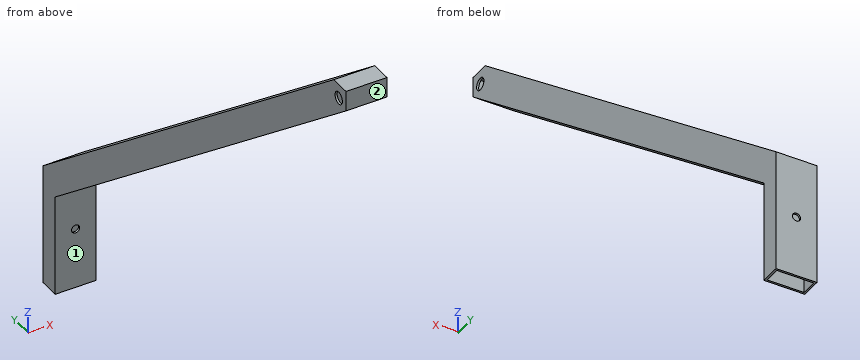
from build123d import *

# Parameters (mm, degrees)
Y_KSEKLIK_EKSTR_ZYON1_DEPTH = 10
BO_ALTMA1_T                 = -1
IZIM2_R                     = 2
KES_EKSTR_ZYON1_DEPTH       = 27
IZIM3_R                     = 3
KES_EKSTR_ZYON2_DEPTH       = 37


with BuildPart() as part:
    # Çizim1 → Yükseklik-Ekstrüzyon1 (new, symmetric)
    with BuildSketch(Plane(origin=(0, 0, 0), x_dir=(0, 0, -1), z_dir=(1, 0, 0))):
        Polygon((0, 0), (-50, 0), (-240, -240), (-250, -240), (-250, -230), (-60, 10), (0, 10), align=None)
    extrude(amount=Y_KSEKLIK_EKSTR_ZYON1_DEPTH, both=True)

    # İç Boşaltma1
    bo_altma1_openings = [part.faces().sort_by_distance(p)[0] for p in [
        (0, 5, 0),
    ]]
    offset(amount=BO_ALTMA1_T, openings=bo_altma1_openings, kind=Kind.INTERSECTION)

    # Çizim2 → Kes-Ekstrüzyon1 (cut)
    with BuildSketch(Plane(origin=(0, 10, 0), x_dir=(1, 0, 0), z_dir=(0, 1, 0))):
        with Locations(Location((0, -30, 0), (0, 0, 270))):
            Circle(IZIM2_R)
    extrude(amount=-KES_EKSTR_ZYON1_DEPTH, mode=Mode.SUBTRACT)

    # Çizim3 → Kes-Ekstrüzyon2 (cut)
    with BuildSketch(Plane.ZY.offset(10)):
        with Locations((243, -234)):
            Circle(IZIM3_R)
    extrude(amount=-KES_EKSTR_ZYON2_DEPTH, mode=Mode.SUBTRACT)


solid = part.part
Can you work these out from the model? Positions are in its coordinate system, mm. Face numbers are marked on the shaded views. A direction names the side the tool comes from. Round coordinates to 2 decimals unless told otherwise and drop trailing zeros. Write each loop counter-clockwise with the first axis right and the second up, starting at its lowest first coordinate (ties: lowest second). Pieces come first, ordered by that corner, then holes. Notation, with made-up numbers: M -12.75,61.25 L 42.25,61.25 A28 cw 42.25,89.25 Z; hole C 45,14 d10. An arc over 180 degrees is marked long. Use CSV: the item, a comma, the result in double quotes.
(1) I need wall thicknesses on line 1 along Y through (x, z) = (6, 50); line 2 along X through (y, z) = (0.35, 30); line 3 along Z through (x, y) = (6.5, -126). Which ranges of each line are inside material? Lowest first, please.
Check values:
line 1,"0 to 1, 9 to 10"
line 2,"-10 to -2, 2 to 10"
line 3,"149.75 to 151.03, 166.39 to 167.67"
(2) Imagine slicing it at A-A (z = 23.5). Write out the boundary of the cut face in (x, y).
Check values:
outline,"M -10,0 L 10,0 L 10,10 L -10,10 Z; hole M -9,1 L 9,1 L 9,9 L -9,9 Z"
(3) Imagine slicing it at B-B (y = -15). Write out the boundary of the cut face in (x, z) (3 decimals), plus the area to 3 significant figures.
Check values:
outline,"M -10,61.875 L 10,61.875 L 10,79.792 L -10,79.792 Z; hole M -9,63.15 L 9,63.15 L 9,78.516 L -9,78.516 Z"
area,"81.7 mm^2"
(4) On a 3-axis mill with a long thin cutter (end or side, diameter ignored), from which of +Z, -Z, +X, -X, +Y, -Y can I reach the whole of each face in a straight line? I mean the marked faces 1 and 2. Say none if no direction works.
Check values:
face 1,"-Z, +X, -X, -Y"
face 2,"+Z, -Z, +X, -X, -Y"
(5) Imagine slicing it at C-C (y = -234). Write out the boundary of the cut face in (x, z).
Check values:
outline,"M -10,235.25 L 10,235.25 L 10,240 L 9,240 L 9,236.53 L -9,236.53 L -9,240 L -10,240 Z; M -10,246 L -9,246 L -9,249 L 9,249 L 9,246 L 10,246 L 10,250 L -10,250 Z"
(6) I'm going to push flat-ended pins straight in: pin 1 (10 mm diameter, centred on x = -3.5, y = -47, fed in from -Z); pin 2 (10 mm diameter, centred on x = 4.5, z = 30, fed in from -Y); pin 3 (3.5 mm diameter, centred on x = 0, z = 30, fed in from -Y); pin 4 (9.5 mm diameter, centred on x = -3, y = -232.5, fed in from -Z). Where does each tip first touch, or does it pass through?
Check values:
pin 1,"z = 83.25"
pin 2,"y = 0"
pin 3,"through"
pin 4,"z = 230.3"
